Input: dimensioned drawing with shaded views. Units: mm. Origin: part minimum x, y, z. Give positions to 0.01 mm unless a question says otherwise; leave off trailing zeros. Loops run counter-clockwise (first coordinate to the right, second up) from the corner with the lowest first, then second, coordinate; pieces in that order, holes last. Notation, with made-up numbers: (-36.75, 28.25) -> (-19.75, 28.25) arc R8 ccw to (-19.75, 42.25) -> close; hole circle Ø9 at (10, 77.5). An arc over 180 degrees is marked (long way). Answer in a Markdown table with one row per item. Add a question column.
1) Line query: line 1 (Z direction, x = 83, y = 0.5) (3 decimals); line 2 (Z direction, x = 33, y = 0.5) (3 decimals); line 3 (X direction, y = 4.25, z = 18.5) (3 decimals). Output: solid intervals per line, ascending. Write a range as from..to.
2) Section query A-A (x = 79.5). Return the cut outline in (y, z) (3 decimals), plus the area to 3 significant figures.
3) Section query B-B (z = 19.5). Return the cut outline in (x, y) (3 decimals).
4) First-contact query: P1, Ø3, axis at x = 98, y = 1.5, coming from the +Z side (3 decimals); P2, Ø3, axis at x = 96.5, y = 2.5, coming from the -Z side (3 decimals); P3, Ø9.5, axis at x = 15.475, z = 15.475, coming from the -Y side; P4, Ø3, axis at y = 2.5, z = 11, coming from the -X side. Flat tips, straight axial feed; report the tip coordinate or a pass-through.
5) Section query D-D (x = 42). Return the cut outline in (y, z) (3 decimals).
6) Section query C-C (y = 5.25). Return the cut outline in (x, z) (3 decimals).
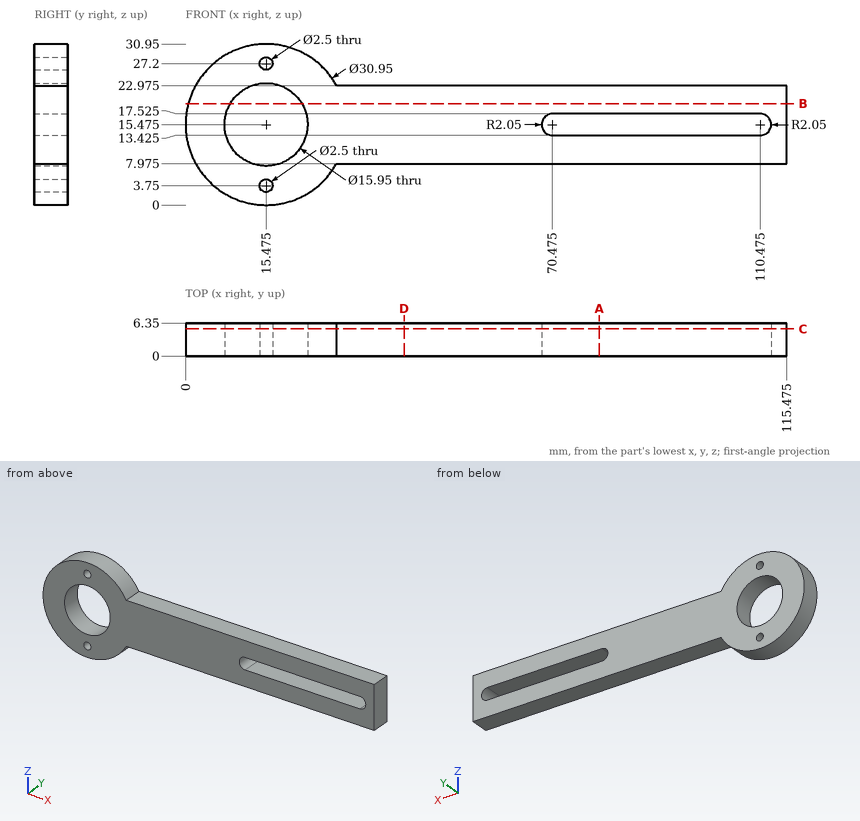
Evaluation:
| question | item | result |
|---|---|---|
| 1 | line 1 | 7.975..13.425, 17.525..22.975 |
| 1 | line 2 | 7.975..22.975 |
| 1 | line 3 | 0.299..8.096, 22.854..115.475 |
| 2 | outline | (0, 7.975) -> (6.35, 7.975) -> (6.35, 13.425) -> (0, 13.425) -> close; (0, 17.525) -> (6.35, 17.525) -> (6.35, 22.975) -> (0, 22.975) -> close |
| 2 | area | 69.2 mm² |
| 3 | outline | (0.533, 0) -> (8.59, 0) -> (8.59, 6.35) -> (0.533, 6.35) -> close; (22.36, 0) -> (115.475, 0) -> (115.475, 6.35) -> (22.36, 6.35) -> close |
| 4 | P1 | z = 22.975 |
| 4 | P2 | z = 7.975 |
| 4 | P3 | through |
| 4 | P4 | x = 0.29 |
| 5 | outline | (0, 7.975) -> (6.35, 7.975) -> (6.35, 22.975) -> (0, 22.975) -> close |
| 6 | outline | (29.011, 7.975) -> (115.475, 7.975) -> (115.475, 22.975) -> (29.011, 22.975) arc R15.475 ccw (long way) to start; hole circle Ø15.95 at (15.475, 15.475); hole circle Ø2.5 at (15.475, 3.75); hole circle Ø2.5 at (15.475, 27.2); hole (70.475, 13.425) -> (110.475, 13.425) arc R2.05 ccw to (110.475, 17.525) -> (70.475, 17.525) arc R2.05 ccw to start |
